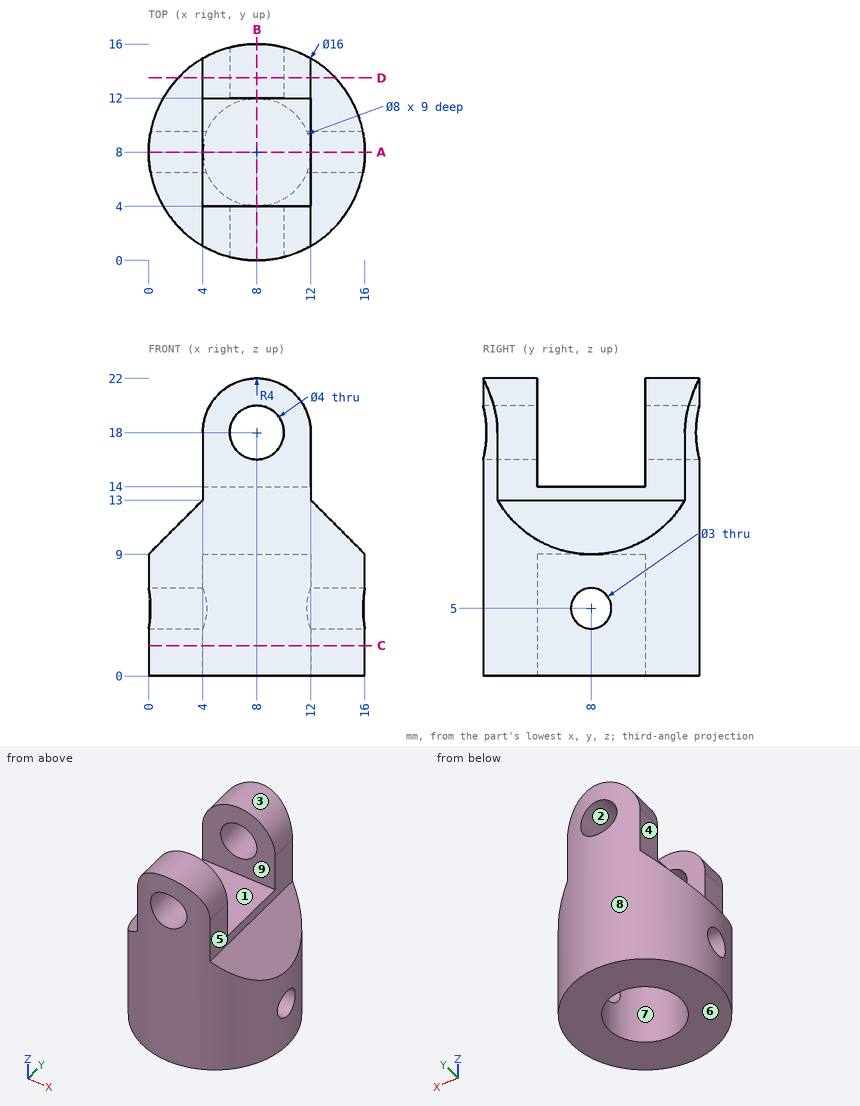
Design review of the part shown in the three views and the two pictorial views. Dimensions are in mm from the part's minimum x, y and z. A direction names the side the tool comes from. Round coordinates to 2 decimals unless told otherwise and drop trailing zeros. Write each loop counter-clockwise with the first axis right and the second up, starting at its lowest first coordinate (ties: lowest second). Pieces come first, ordered by that corner, then holes.
Item 1: Wall thickness on L1, parallel to Y at x = 8, z = 6.25; L2, parallel to Z at x = 8.25, y = 5.5; L3, parallel to Y at x = 2.4, z = 5: over which ranges is each line inside the solid? List them lowest first.
Item 2: For pin 1 Ø4 at (x, y) = (7, 8.5) entering from +Z; pin 2 Ø1.8 at (y, z) = (8, 5) entering from +X; pin 3 Ø6 at (x, y) = (11.5, 6.5) entering from +Z; pin 4 Ø4 at (y, z) = (3.5, 11.5) entering from -X, all flat-tipped, find the tip position at first contact; note any pin that passes through.
Item 3: For the marked faces 1, 2, 3, 4 and 5, list the 3-axis set-ups (+Z, -Z, +X, -X, +Y, -Y) from which the entire face can be reached by the end or side of a thin tool; tool diameter is ignored.
Item 4: Consider section A-A on y = 8. Give the boundary of the cut face in (x, z).
Item 5: Consider section D-D on y = 13.5. Give the boundary of the cut face in (x, z).
Item 6: Consider section B-B on x = 8. Give the boundary of the cut face in (y, z), and give its area (3 significant figures).
Item 7: Draft analysis for pull direction Y (two halves, no side actions). For the marked faces 6, 7, 8 and 9, state which applies: released by +Y, released by -Y, zero draft, split by the parting line, or undercut.
Item 8: Consider section C-C on z = 2.25. Give the boundary of the cut face in (x, y).
Check values:
1. L1: y = 0 to 4, 12 to 16
1. L2: z = 9 to 14
1. L3: y = 2.29 to 6.5, 9.5 to 13.71
2. pin 1: stops at z = 14
2. pin 2: passes through
2. pin 3: stops at z = 21.55
2. pin 4: stops at x = 0.79
3. face 1: +Z, +X, -X
3. face 2: +Y, -Y
3. face 3: +Z, +Y, -Y
3. face 4: +Z, -X, +Y, -Y
3. face 5: +Z, +X, +Y, -Y
4. outline: (0, 0) - (4, 0) - (4, 3.5) - (0, 3.5) - close; (0, 6.5) - (4, 6.5) - (4, 9) - (12, 9) - (12, 6.5) - (16, 6.5) - (16, 9) - (12, 13) - (12, 14) - (4, 14) - (4, 13) - (0, 9) - close; (12, 0) - (16, 0) - (16, 3.5) - (12, 3.5) - close
5. outline: (2.19, 0) - (13.81, 0) - (13.81, 11.19) - (12, 13) - (12, 18) arc R4 ccw to (4, 18) - (4, 13) - (2.19, 11.19) - close; hole circle Ø4 at (8, 18)
6. outline: (0, 0) - (4, 0) - (4, 9) - (12, 9) - (12, 0) - (16, 0) - (16, 16) - (12, 16) - (12, 14) - (4, 14) - (4, 16) - (0, 16) - close; (0, 20) - (4, 20) - (4, 22) - (0, 22) - close; (12, 20) - (16, 20) - (16, 22) - (12, 22) - close
6. area: 184 mm2
7. face 6: zero draft
7. face 7: undercut
7. face 8: split by the parting line
7. face 9: undercut
8. outline: circle Ø16 at (8, 8); hole circle Ø8 at (8, 8)
